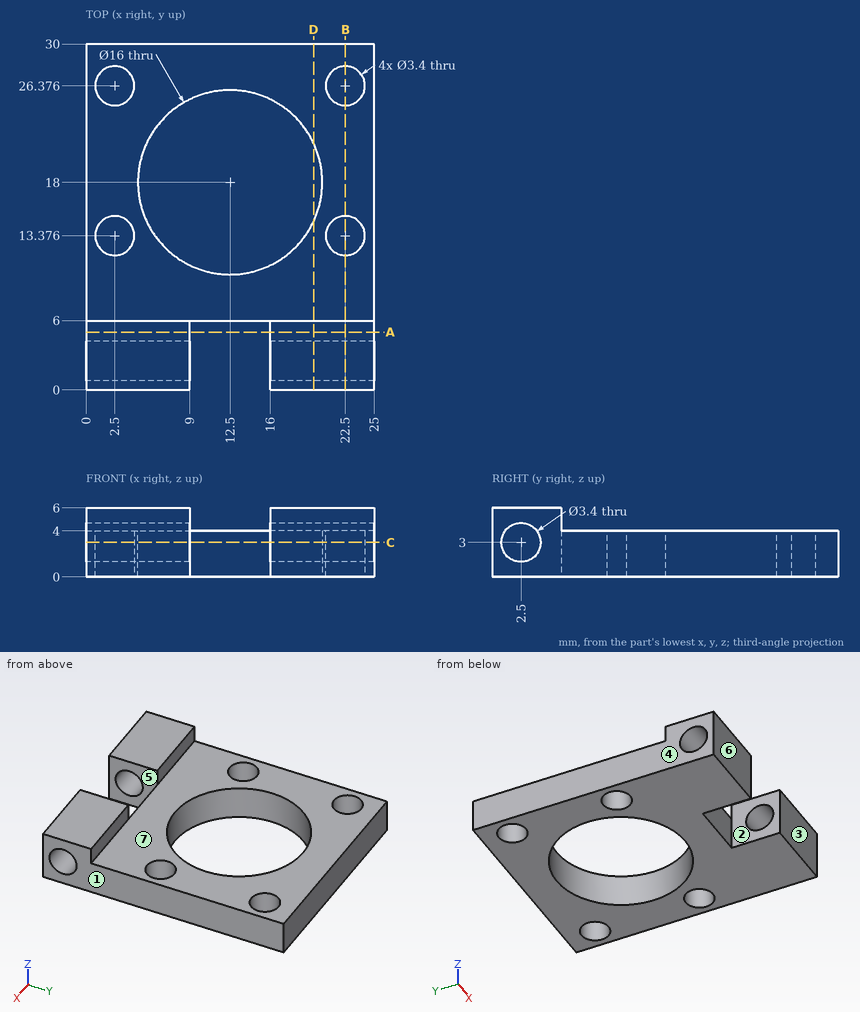
Geometry check sheet. Reference: drawing and pictorial views, mm from the part's lowest x, y, z. A direction names the side the tool comes from. Round coordinates to 2 decimals unless told otherwise and drop trailing zeros. Loops run counter-clockwise (first coordinate to the right, second up) from the corner with the lowest first, then second, coordinate; pieces in that order, holes last. Notation, with made-up numbers: (55, -31.75) - (71, -31.75) arc R12 ccw to (71, -10.75) - close; hole circle Ø4 at (14.25, 79). An arc over 180 degrees is marked (long way). One line per question, with ' | ' between items. Start each with the question number.
1. Cross-section at D-D on x = 19.75. Record the cut outline in (y, z).
2. Scan lines: line 1 (X direction, y = 5.75, z = 0.6); line 2 (Y direction, x = 18.75, z = 3.9) (1 decimal); line 3 (Y direction, x = 2.5, z = 3.1). Record each from-to range of solid material in increasing order. Write a range as [from, to].
3. Depth check by flat-ended pin: pin 1 (3 mm diameter, centred on y = 2.5, z = 4, fed in from -X); pin 2 (4 mm diameter, centred on x = 22.5, y = 13.38, fed in from +Z); pin 3 (1 mm diameter, centred on x = 2.5, z = 5.5, fed in from +Y). Enter the tip coordinate at first touch or a pass-through.
4. Cross-section at B-B on x = 22.5. Record the cut outline in (y, z).
5. Tool access check on the marked faces 5, 6 and 7. Record the directions out of +Z, -Z, +X, -X, +Y, -Y that give a thin tool (end or side, any length) a straight path to the whole face; none if there is none.
6. Draft check along X on the marked faces 1, 2, 3 and 4. Enter one of: released by +X, released by -X, zero draft, split by the parting line, or undercut.
7. Cross-section at A-A on y = 5. Record the cut outline in (x, z), then the cut area to 3 significant figures.
8. Cross-section at C-C on z = 3. Record the cut outline in (x, y).
Taken from the geometry:
1) outline: (0, 0) - (14.62, 0) - (14.62, 4) - (6, 4) - (6, 6) - (0, 6) - close; (21.38, 0) - (30, 0) - (30, 4) - (21.38, 4) - close; hole circle Ø3.4 at (2.5, 3)
2) line 1: [0, 9], [16, 25] | line 2: [0, 1.1], [3.9, 13], [23, 30] | line 3: [0, 0.8], [4.2, 11.68], [15.08, 24.68], [28.08, 30]
3) pin 1: x = 0 | pin 2: z = 4 | pin 3: y = 6
4) outline: (0, 0) - (11.68, 0) - (11.68, 4) - (6, 4) - (6, 6) - (0, 6) - close; (15.08, 0) - (24.68, 0) - (24.68, 4) - (15.08, 4) - close; (28.08, 0) - (30, 0) - (30, 4) - (28.08, 4) - close; hole circle Ø3.4 at (2.5, 3)
5) face 5: +Z, -Z, -Y | face 6: +Z, -Z, +X, -X, -Y | face 7: +Z, +X, -X, +Y
6) face 1: released by +X | face 2: undercut | face 3: zero draft | face 4: released by -X
7) outline: (0, 0) - (9, 0) - (9, 6) - (0, 6) - close; (16, 0) - (25, 0) - (25, 6) - (16, 6) - close | area: 108 mm²
8) outline: (0, 0) - (9, 0) - (9, 0.8) - (0, 0.8) - close; (0, 4.2) - (9, 4.2) - (9, 6) - (16, 6) - (16, 4.2) - (25, 4.2) - (25, 30) - (0, 30) - close; (16, 0) - (25, 0) - (25, 0.8) - (16, 0.8) - close; hole circle Ø3.4 at (2.5, 13.38); hole circle Ø3.4 at (2.5, 26.38); hole circle Ø16 at (12.5, 18); hole circle Ø3.4 at (22.5, 13.38); hole circle Ø3.4 at (22.5, 26.38)
